```python
from build123d import *

# Parameters (mm, degrees)
BOSS_EXTRUDE1_DEPTH = 3
FILLET1_R           = 30


with BuildPart() as part:
    # Sketch1 → Boss-Extrude1 (new body)
    with BuildSketch(Plane.XY):
        Polygon((0, 0), (-0.01, 0), (-0.01, -3), (-10.01, -3), (-10.01, 0), (-18.34, 0), (-18.34, -3), (-28.34, -3), (-28.34, 0), (-36.67, 0), (-36.67, -3), (-46.67, -3), (-46.67, 0), (-55, 0), (-55, -3), (-65, -3), (-65, 0), (-65, 27.612062293), (0, 27.612062293), align=None)
        Polygon((-63.444972674, 23.538741566), (-62.555720301, 25.98194238), (-53.158794094, 22.561740947), (-54.048046466, 20.118540133), align=None, mode=Mode.SUBTRACT)
        Polygon((-45.331154562, 19.712713153), (-35.934228355, 16.29251172), (-36.823480727, 13.849310906), (-46.220406935, 17.269512339), align=None, mode=Mode.SUBTRACT)
        Polygon((-28.106588823, 13.443483926), (-18.709662616, 10.023282493), (-19.598914988, 7.580081679), (-28.995841196, 11.000283112), align=None, mode=Mode.SUBTRACT)
        Polygon((-10.882023084, 7.174254699), (-1.485096877, 3.754053266), (-2.374349249, 1.310852452), (-11.771275457, 4.731053885), align=None, mode=Mode.SUBTRACT)
    extrude(amount=BOSS_EXTRUDE1_DEPTH)

    # Fillet1
    # the kernel refuses this fillet: 30 mm, written as the material it takes off along each edge
    with BuildSketch(Plane(origin=(0, 27.612062293, -74.762028861), x_dir=(-1, 0, 0), z_dir=(0, 0, 1))) as fillet1_piece_1:
        with BuildLine():
            CenterArc((29.904811544, 30), FILLET1_R, 184.565454752, 85.434545248)
            Line((0, 27.612062293), (-0.598096231, 27.564303539))
            ThreePointArc((-0.598096231, 27.564303539), (-0.6, 13.806031146), (-0.6, 0))
            Line((-0.6, 0), (0, -0.6))
            Line((0, -0.6), (29.904811544, -0.6))
            Line((29.904811544, -0.6), (29.904811544, 0))
        make_face()
    extrude(amount=152.524057722, mode=Mode.SUBTRACT)


solid = part.part
```
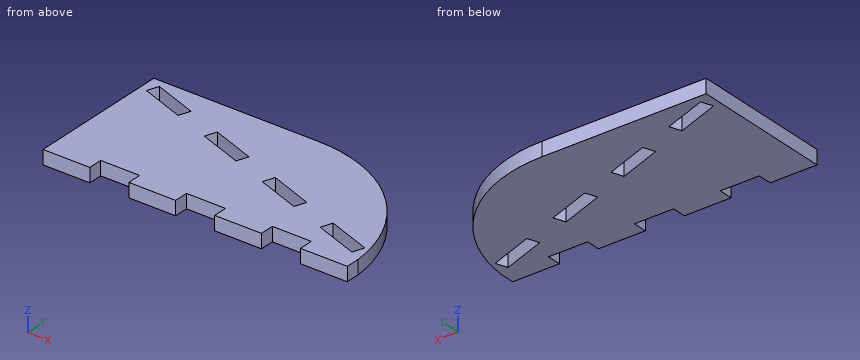
Check sheet for the modelled part. Datum: model origin and axes. Units: mm. Round coordinates to 2 decimals unless told otherwise and drop trailing zeros. Order: outer loops, then holes, each group sorted by start corner. A loop starts at its lowest first (then second) coordinate and runs counter-clockwise, first axis right, second up. Notation, with made-up numbers: (0.25, -15) -> (16.25, -15) arc R21 cw to (16.25, -6) -> close; hole circle Ø2 at (29, 3.25). An arc over 180 degrees is marked (long way). Use CSV: the item, a comma, the result in double quotes.
(1) Depth check by flat-ended pin: pin 1 (1.5 mm diameter, centred on y = -1, z = 2, fed in from +X); pin 2 (1.5 mm diameter, centred on x = -52, z = 2, fed in from -Y). Enter the tip coordinate at first touch or a pass-through.
Worked out:
pin 1,"x = -0.01"
pin 2,"y = 0"
(2) Material ranges on line 1 along X through (y, z) = (-0.5, 0.45); line 2 along Y through (x, z) = (-26, 1.85); line 3 along Y through (x, z) = (-53, 1.45), recorded low to high. Write a range as from..to.
Worked out:
line 1,"-65..-55, -46.67..-36.67, -28.34..-18.34, -10.01..-0.01"
line 2,"-3..9.91, 12.68..27.36"
line 3,"0..27.61"
(3) Cross-section at D-D (x = -33.5). Record the boundary of the cut face in (y, z).
Worked out:
outline,"(0, 0) -> (27.61, 0) -> (27.61, 3) -> (0, 3) -> close"
(4) Cross-section at B-B (y = 15). Record the boundary of the cut face in (x, z), and give its area (3 significant figures).
Worked out:
outline,"(-65, 0) -> (-39.98, 0) -> (-39.98, 3) -> (-65, 3) -> close; (-36.4, 0) -> (-5.46, 0) -> (-5.46, 3) -> (-36.4, 3) -> close"
area,"168 mm²"
(5) Cross-section at C-C (x = -44). Record the boundary of the cut face in (y, z).
Worked out:
outline,"(-3, 0) -> (16.46, 0) -> (16.46, 3) -> (-3, 3) -> close; (19.23, 0) -> (27.61, 0) -> (27.61, 3) -> (19.23, 3) -> close"
(6) Cross-section at A-A (z = 1.15). Count the separate pieces of the cut face and the enclosed holes in it, and give its area (3 significant figures).
Worked out:
separate pieces,"1"
enclosed holes,"4"
area,"1,620 mm²"
